Work out the finished part from the listing and answer in its coordinate system (mm). A direction names the side the tool comes from. Give positions to 0.01 mm unless a question says otherwise; leave off trailing zeros. Loops run counter-clockwise (first coordinate to the right, second up) from the corner with the lowest first, then second, coordinate; pieces in that order, holes last. Notation, with made-up numbers: M 55,-23 L 89,-23 A27 cw 89,10 Z; hole C 70,-3 d2. An arc over 180 degrees is marked long. Use a Markdown table: item, result.
```python
from build123d import *

# Parameters (mm, degrees)
F0_R     = 10
F1_DEPTH = 20
F2_DEPTH = 7
F3_W     = 3
F3_H     = 42
F4_DEPTH = 20.001
F6_DEPTH = 2


with BuildPart() as f1:
    # F0 (on Top) → F1 (new body)
    with BuildSketch(Plane.XY):
        with BuildLine():
            ThreePointArc((-12, 0), (-5.192772811, 10.8182766896), (7.5058517555, 9.3628088427))
            Line((7.5058517555, 9.3628088427), (-12, 25))
            Line((-12, 25), (-12, 0))
        make_face()
        with BuildLine():
            ThreePointArc((7.5058517555, -9.3628088427), (10.8182766896, -5.192772811), (12, 0))
            ThreePointArc((12, 0), (10.8182766896, 5.192772811), (7.5058517555, 9.3628088427))
            ThreePointArc((7.5058517555, 9.3628088427), (-5.192772811, 10.8182766896), (-12, 0))
            ThreePointArc((-12, 0), (-5.192772811, -10.8182766896), (7.5058517555, -9.3628088427))
        make_face()
        Circle(F0_R, mode=Mode.SUBTRACT)
        with BuildLine():
            Line((0, -15.38), (7.5058517555, -9.3628088427))
            ThreePointArc((7.5058517555, -9.3628088427), (-5.192772811, -10.8182766896), (-12, 0))
            Line((-12, 0), (-12, -25))
            Line((-12, -25), (0, -15.38))
        make_face()
    extrude(amount=F1_DEPTH)

    # F2 (add): a face of the model
    f2_faces = [f1.faces().sort_by_distance(p)[0] for p in [
        (-12, 0, 10),
    ]]
    extrude(f2_faces, amount=F2_DEPTH)

    # F3 (on face) → F4 (cut, through all)
    with BuildSketch(Plane.XY.offset(20)):
        with Locations((-15.5, 0)):
            Rectangle(F3_W, F3_H)
    extrude(amount=-F4_DEPTH, mode=Mode.SUBTRACT)

    # F5 (on face) → F6 (cut, through all)
    with BuildSketch(Plane(origin=(-19, 0, 0), x_dir=(0, -1, 0), z_dir=(-1, 0, 0))):
        Polygon((6.5470053838, 0), (9.5470053838, 0), (-2, 20), (-5, 20), align=None)
    extrude(amount=-F6_DEPTH, mode=Mode.SUBTRACT)


solid = f1.part
```
(1) Consider probe 1 along Y at (x, z) = (-15.5, 11); probe 2 along Y at (x, z) = (0, 9.25); probe 3 along X at (y, z) = (-14, 16.25). Determine where each line is inside the solid, lowest interval first. Write a range as [from, to].
Entries:
| item | result |
|---|---|
| probe 1 | y = [-25, -21], [21, 25] |
| probe 2 | y = [-15.38, -10], [10, 15.38] |
| probe 3 | x = [-19, -17], [-14, 1.72] |
(2) The mould has two halves that part along Y. Classify faces 1 (the flat face through (-15, -25, 10)), 2 (the flat face through (-10.2, 0.4, 0)), 3 (the flat face through (-16, 21, 10)): released by +Y, released by -Y, zero draft, split by the parting line, or undercut.
Entries:
| item | result |
|---|---|
| face 1 | released by -Y |
| face 2 | zero draft |
| face 3 | undercut |
(3) A cutting plane is placed at C-C (y = 6). Write down the section's boundary in (x, z), and give its area (3 significant figures).
Entries:
| item | result |
|---|---|
| outline | M -19,0 L -17,0 L -17,20 L -19,20 Z; M -14,0 L -8,0 L -8,20 L -14,20 Z; M 8,0 L 10.39,0 L 10.39,20 L 8,20 Z |
| area | 208 mm² |
(4) A cutting plane is placed at A-A (x = 6). Write down the section's boundary in (y, z).
Entries:
| item | result |
|---|---|
| outline | M -10.57,0 L -8,0 L -8,20 L -10.57,20 Z; M 8,0 L 10.57,0 L 10.57,20 L 8,20 Z |
(5) A cutting plane is placed at D-D (z = 9.25). Write down the section's boundary in (x, y).
Entries:
| item | result |
|---|---|
| outline | M -19,-25 L -12,-25 L 7.51,-9.36 A12 ccw 7.51,9.36 L -12,25 L -19,25 L -19,-1.21 L -17,-1.21 L -17,21 L -14,21 L -14,-21 L -17,-21 L -17,-4.21 L -19,-4.21 Z; hole C 0,0 d20 |
(6) Which of the six approach directions +Z, -Z, +X, -X, +Y, -Y give full straight-line access (tool end or side, diameter ignored) to faces 4 (the flat face through (-15, 25, 10)), 5 (the flat face through (-17, -12, 10)), 6 (the flat face through (-18.014, -3.854, 9.86))?
Entries:
| item | result |
|---|---|
| face 4 | +Z, -Z, +X, -X, +Y |
| face 5 | +Z, -Z |
| face 6 | -X |
(7) A cutting plane is placed at B-B (y = -18.5). Write down the section's boundary in (x, z), and give its area (3 significant figures).
Entries:
| item | result |
|---|---|
| outline | M -19,0 L -17,0 L -17,20 L -19,20 Z; M -14,0 L -3.89,0 L -3.89,20 L -14,20 Z |
| area | 242 mm² |
(8) Given P1, Ø12, axis at x = 8.5, z = 4.5, coming from the -Y side; P2, Ø12, axis at x = 0.5, z = 4.5, coming from the -Y side; P3, Ø12, axis at y = -11.5, z = 6, coming from the +X side, each flat-ended and moving along its own axis, determine where each tip first touches the part or whether it passes through.
Entries:
| item | result |
|---|---|
| P1 | stops at y = -13.38 |
| P2 | stops at y = -19.79 |
| P3 | stops at x = 10.67 |
